Solid Edge part; units mm, degrees
sketch "Sketch1" plane through (0, 0, 0) normal (0, -1, 0) x (1, 0, 0)
  circle A0 centre (0, 0) radius 16
extrude "Protrusion1" add sketch "Sketch1" along normal mid plane 11
hole "Bohrung_1" at (0, -5.5, 0) direction (0, 1, 0) diameter 20 end up to next
fillet "Verrundung_1" radius 0.5 4 edges at (-16, -5.5, 0) (-16, 5.5, 0) (-10, -5.5, 0) (0, 5.5, -10)
sketch "Sketch2" plane through (0, -5.5, 0) normal (0, -1, 0) x (1, 0, 0)
  circle A0 centre (0, 0) radius 11
  circle A1 centre (0, 0) radius 15
extrude "Extrusionsausschnitt_1" cut sketch "Sketch2" along normal mid plane 1
mirror "Mirror1" about plane through (0, 0, 0) normal (0, -1, 0) of "Extrusionsausschnitt_1"
properties material "Aluminium, 1060"
Geometry check sheet. Reference: the model listing, model coordinates, mm. A direction names the side the tool comes from. Coordinates: 2 decimals unless noted, no trailing zeros. Order: outer loops, then holes, each group sorted by start corner. A loop starts at its lowest first (then second) coordinate and runs counter-clockwise, first axis right, second up.
Item 1: Section check C-C (y = -3). Enter the section's corners in (x, z), plus the area to 3 significant figures.
Item 2: Tool access check on faces 1 (the flat face through (10, 5, -5)), 2 (the flat face through (-4, -5.5, -10)), 3 (the flat face through (10, -5, 5)). Record the directions out of +Z, -Z, +X, -X, +Y, -Y that give a thin tool (end or side, any length) a straight path to the whole face; none if there is none.
Item 3: Scan lines: line 1 along Z through (x, y) = (0, 2.25); line 2 along Y through (x, z) = (5, 13); line 3 along Z through (x, y) = (-8.5, -1.5). Record each from-to range of solid material in increasing order.
Item 4: Depth check by flat-ended pin: pin 1 (9 mm diameter, centred on x = -7.5, z = -1, fed in from -Y); pin 2 (4 mm diameter, centred on x = -8, y = -2, fed in from -Z); pin 3 (1.5 mm diameter, centred on x = -8, y = 2, fed in from -Z); pin 4 (1.5 mm diameter, centred on y = -1.5, z = -2, fed in from +X). Enter the tip coordinate at first touch or a pass-through.
Item 5: Mould release check, pull along X, two halves, no side actions. Record for faces 4 (the cylindrical face through (-2.38, -5.25, -10.74)), 5 (the cylindrical face through (-3.47, 0.07, 15.62)), 6 (the flat face through (13, 5.5, 8)), 7 (the cylindrical face through (-2.38, 5.25, 10.74)): released by +X, released by -X, zero draft, split by the parting line, or undercut.
Check sheet entries:
1. outline: circle Ø32 at (0, 0); hole circle Ø20 at (0, 0)
1. area: 490 mm2
2. face 1: +Y
2. face 2: +Z, -Z, +X, -X, -Y
2. face 3: -Y
3. line 1: z = -16 to -10, 10 to 16
3. line 2: y = -5 to 5
3. line 3: z = -13.56 to -5.27, 5.27 to 13.56
4. pin 1: stops at y = -5.5
4. pin 2: stops at z = -14.83
4. pin 3: stops at z = -14.26
4. pin 4: stops at x = 15.95
5. face 4: undercut
5. face 5: split by the parting line
5. face 6: zero draft
5. face 7: undercut
